Read the model definition and answer for the solid it produces. Units are mm, in the model's axes. Face numbers are marked on the shaded views. Give positions to 0.01 mm unless a question says otherwise; leave off trailing zeros. Order: outer loops, then holes, each group sorted by start corner. A loop starts at its lowest first (then second) coordinate and runs counter-clockwise, first axis right, second up. Notation, with made-up numbers: (-34.75, 7.25) - (-21.75, 7.25) arc R21 ccw to (-21.75, 28.25) - close; hole circle Ø2 at (23.25, 55). An arc over 180 degrees is marked (long way). Write item = value, one per line.
```python
from build123d import *

# Parameters (mm, degrees)
SKETCH1_W           = 91
SKETCH1_H           = 55.5
BOSS_EXTRUDE1_DEPTH = 5
FILLET1_R           = 1
FILLET2_R           = 1
SKETCH3_R           = 2.5
SKETCH3_R_2         = 4.5
SKETCH3_R_3         = 3.5
CUT_EXTRUDE6_DEPTH  = 5
SHELL3_START        = 2
SHELL3_OUTLINE_R    = 5.5
SHELL3_OUTLINE_R_2  = 6.5
SHELL3_DEPTH        = 3


# Read off the part's stored shape, not the designer's step: Shell3
with BuildPart() as part:
    # Sketch1 → Boss-Extrude1 (new body)
    with BuildSketch(Plane.XY):
        with Locations((45.5, -27.75)):
            Rectangle(SKETCH1_W, SKETCH1_H)
    extrude(amount=BOSS_EXTRUDE1_DEPTH)

    # Fillet1
    fillet1_edges = [part.edges().sort_by_distance(p)[0] for p in [
        (0, -27.75, 5),
        (45.5, -55.5, 0),
        (0, -27.75, 0),
        (45.5, -55.5, 5),
        (0, 0, 2.5),
        (91, -55.5, 2.5),
        (0, -55.5, 2.5),
    ]]
    fillet(fillet1_edges, radius=FILLET1_R)

    # Fillet2
    # the kernel refuses this fillet: 1 mm, written as the material it takes off along each edge
    with BuildSketch(Plane(origin=(90, -54.5, 4), x_dir=(0, 0, 1), z_dir=(1, 0, 0))) as fillet2_piece_1_section:
        Polygon((0, 0), (FILLET2_R, 0), (FILLET2_R, FILLET2_R), (0, FILLET2_R), align=None)
    fillet2_piece_1 = extrude(amount=FILLET2_R, mode=Mode.PRIVATE)
    fillet2_piece_1 = fillet2_piece_1 - Plane(origin=(90, -54.5, 4), x_dir=(0, 0.7071067811865475, -0.7071067811865475), z_dir=(1, 0, 0)) * Sphere(FILLET2_R, mode=Mode.PRIVATE)
    add(fillet2_piece_1, mode=Mode.SUBTRACT)
    with BuildSketch(Plane(origin=(90, -54.5, 1), x_dir=(1, 0, 0), z_dir=(0, 0, -1))) as fillet2_piece_2_section:
        Polygon((0, 0), (FILLET2_R, 0), (FILLET2_R, FILLET2_R), (0, FILLET2_R), align=None)
    fillet2_piece_2 = extrude(amount=FILLET2_R, mode=Mode.PRIVATE)
    fillet2_piece_2 = fillet2_piece_2 - Plane(origin=(90, -54.5, 1), x_dir=(-0.7071067811865476, 0.7071067811865475, 0), z_dir=(0, 0, -1)) * Sphere(FILLET2_R, mode=Mode.PRIVATE)
    add(fillet2_piece_2, mode=Mode.SUBTRACT)
    with BuildSketch(Plane(origin=(1, -1, 4), x_dir=(0, 0, 1), z_dir=(0, 1, 0))) as fillet2_piece_3_section:
        Polygon((0, 0), (FILLET2_R, 0), (FILLET2_R, -FILLET2_R), (0, -FILLET2_R), align=None)
    fillet2_piece_3 = extrude(amount=FILLET2_R, mode=Mode.PRIVATE)
    fillet2_piece_3 = fillet2_piece_3 - Plane(origin=(1, -1, 4), x_dir=(0.7071067811865475, 0, -0.7071067811865475), z_dir=(0, 1, 0)) * Sphere(FILLET2_R, mode=Mode.PRIVATE)
    add(fillet2_piece_3, mode=Mode.SUBTRACT)
    with BuildSketch(Plane(origin=(1, -1, 1), x_dir=(0, 0, -1), z_dir=(0, 1, 0))) as fillet2_piece_4_section:
        Polygon((0, 0), (FILLET2_R, 0), (FILLET2_R, FILLET2_R), (0, FILLET2_R), align=None)
    fillet2_piece_4 = extrude(amount=FILLET2_R, mode=Mode.PRIVATE)
    fillet2_piece_4 = fillet2_piece_4 - Plane(origin=(1, -1, 1), x_dir=(0.7071067811865475, 0, 0.7071067811865475), z_dir=(0, 1, 0)) * Sphere(FILLET2_R, mode=Mode.PRIVATE)
    add(fillet2_piece_4, mode=Mode.SUBTRACT)
    with BuildSketch(Plane(origin=(90, -1, 4), x_dir=(1, 0, 0), z_dir=(0, 1, 0))) as fillet2_piece_5_section:
        Polygon((0, 0), (FILLET2_R, 0), (FILLET2_R, -FILLET2_R), (0, -FILLET2_R), align=None)
    fillet2_piece_5 = extrude(amount=FILLET2_R, mode=Mode.PRIVATE)
    fillet2_piece_5 = fillet2_piece_5 - Plane(origin=(90, -1, 4), x_dir=(-0.7071067811865475, 0, -0.7071067811865475), z_dir=(0, 1, 0)) * Sphere(FILLET2_R, mode=Mode.PRIVATE)
    add(fillet2_piece_5, mode=Mode.SUBTRACT)
    with BuildSketch(Plane(origin=(90, -1, 1), x_dir=(0, 0, -1), z_dir=(0, 1, 0))) as fillet2_piece_6_section:
        Polygon((0, 0), (FILLET2_R, 0), (FILLET2_R, -FILLET2_R), (0, -FILLET2_R), align=None)
    fillet2_piece_6 = extrude(amount=FILLET2_R, mode=Mode.PRIVATE)
    fillet2_piece_6 = fillet2_piece_6 - Plane(origin=(90, -1, 1), x_dir=(-0.7071067811865475, 0, 0.7071067811865475), z_dir=(0, 1, 0)) * Sphere(FILLET2_R, mode=Mode.PRIVATE)
    add(fillet2_piece_6, mode=Mode.SUBTRACT)
    with BuildSketch(Plane(origin=(91, -1, 5), x_dir=(0, 0, -1), z_dir=(0, -1, 0)), Plane(origin=(91, -1, 0), x_dir=(-1, 0, 0), z_dir=(0, -1, 0))) as fillet2_piece_7:
        with BuildLine():
            CenterArc((FILLET2_R, -FILLET2_R), FILLET2_R, 90, 90)
            Line((0, -FILLET2_R), (0, 0))
            Line((0, 0), (FILLET2_R, 0))
        make_face()
    extrude(amount=53.5, mode=Mode.SUBTRACT)
    with BuildSketch(Plane(origin=(1, 0, 0), x_dir=(0, 0, 1), z_dir=(1, 0, 0))) as fillet2_piece_8:
        with BuildLine():
            CenterArc((FILLET2_R, FILLET2_R), FILLET2_R, 180, 90)
            Line((0, FILLET2_R), (0, 0))
            Line((0, 0), (FILLET2_R, 0))
        make_face()
    extrude(amount=89, mode=Mode.SUBTRACT)
    with BuildSketch(Plane(origin=(1, 0, 5), x_dir=(0, 0, -1), z_dir=(1, 0, 0))) as fillet2_piece_9:
        with BuildLine():
            CenterArc((FILLET2_R, -FILLET2_R), FILLET2_R, 90, 90)
            Line((0, -FILLET2_R), (0, 0))
            Line((0, 0), (FILLET2_R, 0))
        make_face()
    extrude(amount=89, mode=Mode.SUBTRACT)
    with BuildSketch(Plane(origin=(91, 0, 1), x_dir=(-1, 0, 0), z_dir=(0, 0, 1))) as fillet2_piece_10:
        with BuildLine():
            CenterArc((FILLET2_R, FILLET2_R), FILLET2_R, 180, 90)
            Line((0, FILLET2_R), (0, 0))
            Line((0, 0), (FILLET2_R, 0))
        make_face()
    extrude(amount=3, mode=Mode.SUBTRACT)

    # Sketch3 → Cut-Extrude6 (cut)
    with BuildSketch(Plane(origin=(0, 0, 0), x_dir=(-1, 0, 0), z_dir=(0, 0, -1))):
        with Locations((-4.5, -51)):
            Circle(SKETCH3_R)
        with Locations((-47.337477188, -19.094515349)):
            Circle(SKETCH3_R_2)
        with Locations((-4.5, -4.5)):
            Circle(SKETCH3_R)
        with Locations((-54.590676617, -28.862157246)):
            Circle(SKETCH3_R_3)
        with Locations((-86.5, -4.5)):
            Circle(SKETCH3_R)
        with Locations((-86.5, -51)):
            Circle(SKETCH3_R)
    extrude(amount=-CUT_EXTRUDE6_DEPTH, mode=Mode.SUBTRACT)

    # Shell3 outline → Shell3 (cut)
    with BuildSketch(Plane.XY.offset(SHELL3_START)):
        with BuildLine():
            Line((2, -8.241657387), (2, -47.258342613))
            ThreePointArc((2, -47.258342613), (7.681980515, -47.818019485), (8.241657387, -53.5))
            Line((8.241657387, -53.5), (82.758342613, -53.5))
            ThreePointArc((82.758342613, -53.5), (83.318019485, -47.818019485), (89, -47.258342613))
            Line((89, -47.258342613), (89, -8.241657387))
            ThreePointArc((89, -8.241657387), (83.318019485, -7.681980515), (82.758342613, -2))
            Line((82.758342613, -2), (8.241657387, -2))
            ThreePointArc((8.241657387, -2), (7.681980515, -7.681980515), (2, -8.241657387))
        make_face()
        with Locations((54.590676617, -28.862157246)):
            Circle(SHELL3_OUTLINE_R, mode=Mode.SUBTRACT)
        with Locations((47.337477188, -19.094515349)):
            Circle(SHELL3_OUTLINE_R_2, mode=Mode.SUBTRACT)
    extrude(amount=SHELL3_DEPTH, mode=Mode.SUBTRACT)


solid = part.part
```
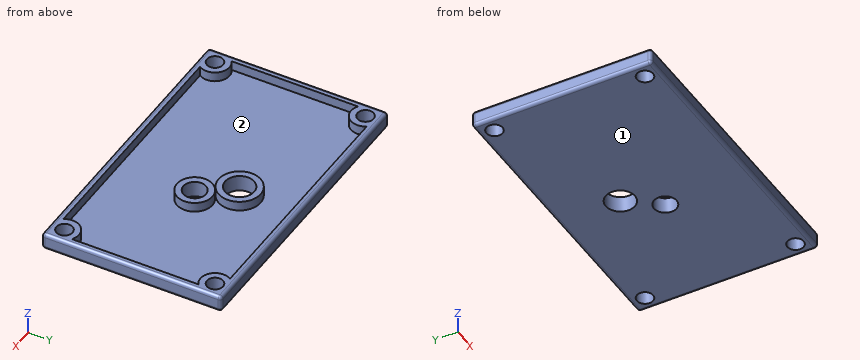
1. A flat-ended cylindrical pin translates along its axis: pin 1 (4.5 mm diameter, centred on x = 4.5, y = -4.5, fed in from -Z). Find the tip coordinate at first contact, or state that the pin passes through.
Recorded:
pin_1 = through
2. Straight lines are drawn through the part: L1, parallel to Y at x = 86.5, z = 3.2; L2, parallel to X at y = -19.5, z = 1.55; L3, parallel to Y at x = 75.5, z = 2.25. For each, find the intervals that lie inside material, in ascending order. Write a range as [from, to].
Recorded:
L1 = [-55.5, -53.5], [-48.5, -46.5], [-9, -7], [-2, 0]
L2 = [0, 42.86], [51.82, 91]
L3 = [-55.5, -53.5], [-2, 0]
3. Section B-B (y = -51) is taken. Determine the outline of the cut face in (x, z), and give its area (3 significant figures).
Recorded:
outline = (0, 1) arc R1 ccw to (1, 0) - (2, 0) - (2, 5) - (1, 5) arc R1 ccw to (0, 4) - close; (7, 0) - (84, 0) - (84, 5) - (82, 5) - (82, 2) - (9, 2) - (9, 5) - (7, 5) - close; (89, 0) - (90, 0) arc R1 ccw to (91, 1) - (91, 4) arc R1 ccw to (90, 5) - (89, 5) - close
area = 185 mm^2
4. Determine the mould class of the marked faces 1 and 2 for opening direction X: +X half, -X half, draft (parallel to the pull), parting line (faces both ways), or undercut.
Recorded:
face_1 = draft
face_2 = undercut
5. Section D-D (y = -38) is taken. Determine the outline of the cut face in (x, z).
Recorded:
outline = (0, 1) arc R1 ccw to (1, 0) - (90, 0) arc R1 ccw to (91, 1) - (91, 4) arc R1 ccw to (90, 5) - (89, 5) - (89, 2) - (2, 2) - (2, 5) - (1, 5) arc R1 ccw to (0, 4) - close
6. Section C-C (z = 3) is taken. Count the separate pieces of the cut face and the enclosed holes in it, and give its area (3 significant figures).
Recorded:
separate_pieces = 3
enclosed_holes = 7
area = 790 mm^2
7. Section A-A (x = 4.5) is taken. Determine the outline of the cut face in (y, z), and give its area (3 significant figures).
Recorded:
outline = (-55.5, 1) arc R1 ccw to (-54.5, 0) - (-53.5, 0) - (-53.5, 5) - (-54.5, 5) arc R1 ccw to (-55.5, 4) - close; (-48.5, 0) - (-7, 0) - (-7, 5) - (-9, 5) - (-9, 2) - (-46.5, 2) - (-46.5, 5) - (-48.5, 5) - close; (-2, 0) - (-1, 0) arc R1 ccw to (0, 1) - (0, 4) arc R1 ccw to (-1, 5) - (-2, 5) - close
area = 114 mm^2
